Verification items for the finished model (mm, model axes). A direction names the side the tool comes from. Give positions to 0.01 mm unless a question says otherwise; leave off trailing zeros. Order: outer loops, then holes, each group sorted by start corner. A loop starts at its lowest first (then second) coordinate and runs counter-clockwise, first axis right, second up. Notation, with made-up numbers: (-20, 25) - (7, 25) arc R12 ccw to (7, 32) - close; hole circle Ø7 at (74.5, 17.25). An arc over 180 degrees is marked (long way). Answer as a JSON object with one key per item and string values. Group by question number.
(1) Mould release check, pull along X, two halves, no side actions. Record for faces 1 (the face through (14.48, -1.01, 0.8)), 2 (the face through (31, -15.081, -13)), 3 (the face through (-19.05, -3, 1)), 4 (the face through (31.75, -3, -23)): +X half, -X half, draft (parallel to the pull), parting line (faces both ways), or undercut.
(2) Access from +Z, -Z, +X, -X, +Y, -Y to the whole of each face (thin tool, end or side, straight path). Record for faces 5 (the face through (30.162, -3, -24)), 6 (the face through (30.945, -3.59, -38.427)).
(3) Section check B-B (y = -3.5). Record the boundary of the cut face in (x, z).
(4) Thickness scan on line 1 (Z direction, x = 21, y = 5.25); line 2 (X direction, y = 6.75, z = -40.5). Record the ranges inside material, lowest first.
(5) Depth check by flat-ended pin: pin 1 Ø7 at (y, z) = (-2.38, -40.32) entering from +X; pin 2 Ø6 at (x, y) = (21, 2.5) entering from -Z. Enter the tip coordinate at first touch or a pass-through.
(6) Section check A-A (x = 12.7). Record the boundary of the cut face in (y, z).
(7) Section check D-D (z = -10.5). Record the boundary of the cut face in (x, y), then the cut area to 3 significant figures.
(8) Section check C-C (y = 7.75). Record the boundary of the cut face in (x, z).
```python
from build123d import *

# Parameters (mm, degrees)
F0_W     = 50.8
F0_H     = 25.4
F1_DEPTH = 1.5875
F2_D     = 4.4958
F3_W     = 25.4
F3_H     = 50.8
F4_DEPTH = 1.5875
F5_D     = 4.4958


# Not quite as in the source:
# - a length typed as a fraction of an inch, garbled in the dataset ("3 / 203.2 mm" for 3/8 in), is restored


with BuildPart() as f1:
    # F0 (on Top) → F1 (new body)
    with BuildSketch(Plane.XY):
        with Locations((6.3499998267, -2.3812473148)):
            Rectangle(F0_W, F0_H)
    extrude(amount=F1_DEPTH)

    # F2 (through all)
    with Locations(Plane(origin=(0, 0, 0), x_dir=(1, 0, 0), z_dir=(0, 0, -1))):
        with Locations((-10.1600001733, 2.3812473148), (12.6999998267, 2.3812473148)):
            Hole(F2_D / 2)

    # F3 (on face) → F4 (join)
    with BuildSketch(Plane.YZ.offset(31.7499998267)):
        with Locations((-2.3812473148, -23.8125)):
            Rectangle(F3_W, F3_H)
    extrude(amount=-F4_DEPTH)

    # F5 (through all)
    with Locations(Plane.YZ.offset(31.7499998267)):
        with Locations((-2.3812473148, -17.4625), (-2.3812473148, -40.3225)):
            Hole(F5_D / 2)


solid = f1.part
```
Solutions:
{
 "1": {"face 1": "undercut", "face 2": "draft", "face 3": "-X half", "face 4": "+X half"},
 "2": {"face 5": "-Z, -X, +Y, -Y", "face 6": "+X, -X"},
 "3": {"outline": "(-19.05, 0) - (-12.11, 0) - (-12.11, 1.59) - (-19.05, 1.59) - close; (-8.21, 0) - (10.75, 0) - (10.75, 1.59) - (-8.21, 1.59) - close; (14.65, 0) - (30.16, 0) - (30.16, -15.51) - (31.75, -15.51) - (31.75, 1.59) - (14.65, 1.59) - close; (30.16, -49.21) - (31.75, -49.21) - (31.75, -42.27) - (30.16, -42.27) - close; (30.16, -38.37) - (31.75, -38.37) - (31.75, -19.41) - (30.16, -19.41) - close"},
 "4": {"line 1": "z = 0 to 1.59", "line 2": "x = 30.16 to 31.75"},
 "5": {"pin 1": "stops at x = 31.75", "pin 2": "stops at z = 0"},
 "6": {"outline": "(-15.08, 0) - (-4.63, 0) - (-4.63, 1.59) - (-15.08, 1.59) - close; (-0.13, 0) - (10.32, 0) - (10.32, 1.59) - (-0.13, 1.59) - close"},
 "7": {"outline": "(30.16, -15.08) - (31.75, -15.08) - (31.75, 10.32) - (30.16, 10.32) - close", "area": "40.3 mm2"},
 "8": {"outline": "(-19.05, 0) - (30.16, 0) - (30.16, -49.21) - (31.75, -49.21) - (31.75, 1.59) - (-19.05, 1.59) - close"}
}
